Here's how the part is built. I have some questions about the finished solid (model axes, mm). A direction names the side the tool comes from. Give positions to 0.01 mm unless a question says otherwise; leave off trailing zeros. Write each loop counter-clockwise with the first axis right and the second up, starting at its lowest first coordinate (ties: lowest second). Pieces come first, ordered by that corner, then holes. Notation, with made-up numbers: (35.25, -20) - (61.25, -20) arc R18 cw to (61.25, 12) - close; hole circle Ø10 at (62.25, 26.25). An arc over 180 degrees is marked (long way). Write each question's results on one line, items separated by ' | '. Start each with the question number.
Item 1: Suppose I cut it at A-A on y = 39. List the corners of the cut face in (x, z) for me, then the cut area to 3 significant figures.
Item 2: Will these pins go through, and if not, where does the flat tip stop? P1, Ø4, axis at x = 13, y = 30, coming from the -Z side; P2, Ø2, axis at y = 43.5, z = -6, coming from the +X side; P3, Ø6.5, axis at y = 21.5, z = 0, coming from the +X side.
Item 3: Which directions (+Z, -Z, +X, -X, +Y, -Y) give clear straight access to the entire face, cutting with the end or side of a thin tool? Please do faces 1 (the flat face through (0, 80, 0)), 2 (the flat face through (13, 30, -4)).
Item 4: We'd pull the mould along Z, two halves only. Please class faces 3 (the flat face through (13, 30, 4)), 4 (the flat face through (0, 0, 0)), 5 (the conical face through (-13.115, 0.125, -0.528)): +Z half, -Z half, draft (parallel to the pull), parting line (faces both ways), or undercut.
Item 5: Please list where these lines run through material, in increasing order: line 1 along X through (y, z) = (43, 7.5); line 2 along Z through (x, y) = (13, 13.5).
```python
from build123d import *

# Parameters (mm, degrees)
BOSS_EXTRUDE1_DEPTH = 80
CUT_EXTRUDE1_DEPTH  = 60
FILLET1_R           = 3
CHAMFER1_SIZE       = 2


with BuildPart() as part:
    # Sketch1 → Boss-Extrude1 (new body)
    with BuildSketch(Plane(origin=(0, 0, 0), x_dir=(1, 0, 0), z_dir=(0, 1, 0))):
        with BuildLine():
            Line((14.456832295, 4), (11, 4))
            Line((11, 4), (11, -4))
            Line((11, -4), (14.456832295, -4))
            ThreePointArc((14.456832295, -4), (14.863587797, -2.018355219), (15, 0))
            ThreePointArc((15, 0), (14.863587797, 2.018355219), (14.456832295, 4))
        make_face()
        with BuildLine():
            Line((11, -4), (11, 4))
            Line((11, 4), (14.456832295, 4))
            ThreePointArc((14.456832295, 4), (-15, 0), (14.456832295, -4))
            Line((14.456832295, -4), (11, -4))
        make_face()
    extrude(amount=BOSS_EXTRUDE1_DEPTH)

    # Sketch1_3 → Cut-Extrude1 (cut)
    with BuildSketch(Plane(origin=(0, 0, 0), x_dir=(1, 0, 0), z_dir=(0, 1, 0))):
        Polygon((94.562608629, 4), (14.456832295, 4), (11, 4), (11, -4), (14.456832295, -4), (94.562608629, -4), (254.774161296, -4), (254.774161296, 4), align=None)
    extrude(amount=CUT_EXTRUDE1_DEPTH, mode=Mode.SUBTRACT)

    # Fillet1
    fillet1_edges = [part.edges().sort_by_distance(p)[0] for p in [
        (11, 60, 0),
    ]]
    fillet(fillet1_edges, radius=FILLET1_R)

    # Chamfer1
    chamfer1_edges = [part.edges().sort_by_distance(p)[0] for p in [
        (-15, 0, 0),
    ]]
    chamfer(chamfer1_edges, length=CHAMFER1_SIZE)


solid = part.part
```
Checked values:
1) outline: (11, -4) - (11, 4) - (14.46, 4) arc R15 ccw (long way) to (14.46, -4) - close | area: 676 mm^2
2) P1: stops at z = -10.2 | P2: stops at x = 14.14 | P3: stops at x = 11
3) face 1: +Z, -Z, +X, -X, +Y | face 2: +X, -Y
4) face 3: undercut | face 4: draft | face 5: parting line
5) line 1: x = -12.99 to 12.99 | line 2: z = -7.48 to -4, 4 to 7.48
